```python
from build123d import *

# Parameters (mm, degrees)
SKETCH_2_OUTSIDE_W  = 32.184
SKETCH_2_OUTSIDE_H  = 32.184
CUT_EXTRUDE_1_DEPTH = 59.533728738
CHAMFER_1_SIZE      = 1


with BuildPart() as part:
    # Эскиз1 → Повернуть1 (revolve)
    with BuildSketch(Plane.XY, mode=Mode.PRIVATE) as revolve_1_sk:
        Polygon((-6.58, 0), (-6.58, 8.85), (0, 8.85), (0, 7.448974596), (0.6, 7.288205081), (0.6, 5), (50.6, 5), (50.6, 0), align=None)
    revolve(revolve_1_sk.sketch.rotate(Axis((-1000, 0, 0), (1, 0, 0)), 90), axis=Axis((-1000, 0, 0), (1, 0, 0)))

    # Эскиз2 outside → Вырез-Вытянуть1 (cut, through all)
    with BuildSketch(Plane.ZY.offset(6.58)):
        Rectangle(SKETCH_2_OUTSIDE_W, SKETCH_2_OUTSIDE_H)
        Polygon((0, -8.85), (7.664324823, -4.425), (7.664324823, 4.425), (0, 8.85), (-7.664324823, 4.425), (-7.664324823, -4.425), align=None, mode=Mode.SUBTRACT)
    extrude(amount=-CUT_EXTRUDE_1_DEPTH, mode=Mode.SUBTRACT)

    # Эскиз4 → Вырез-Повернуть1 (revolve, cut)
    with BuildSketch(Plane.XY):
        Polygon((-6.58, 8.075), (-6.297923068, 8.85), (-6.58, 8.85), align=None)
    revolve(axis=Axis((-1000, 0, 0), (1, 0, 0)), mode=Mode.SUBTRACT)

    # Фаска1
    chamfer_1_edges = [part.edges().sort_by_distance(p)[0] for p in [
        (50.6, 0, -5),
    ]]
    chamfer(chamfer_1_edges, length=CHAMFER_1_SIZE)


solid = part.part
```
Geometry: final body of the model. Coordinates: model frame, mm. A direction names the side the tool comes from. Coordinates: 2 decimals unless noted, no trailing zeros. Order: outer loops, then holes, each group sorted by start corner. A loop starts at its lowest first (then second) coordinate and runs counter-clockwise, first axis right, second up. Notation, with made-up numbers: M 36,-39.5 L 83,-39.5 A18 cw 83,-35.5 Z; hole C 44.25,84 d3. An arc over 180 degrees is marked long. Answer in a Markdown table with one row per item. Add a question column.
Q1. Reachability of faces 1 (the flat face through (0.6, 5, -2)), 2 (the conical face through (-6.5, -4.13, 7.2)) from +Z, -Z, +X, -X, +Y, -Y: full face, straight path, thin tool, end or side. Return the list, or none.
Q2. Section query A-A on y = 0. Return the cut outline in (x, z).
Q3. Contact query for flat-ended pins moving along their axis: P1, Ø5, axis at x = 27, z = 6, coming from the +Y side; P2, Ø10, axis at x = 32.5, y = 3.5, coming from the -Z side; P3, Ø10, axis at x = 20.5, y = 4, coming from the +Z side. Output: stop coordinate, or through.
Q4. Section query B-B on x = 8.5. Return the cut outline in (y, z), and give its area (3 significant figures).
Q5. Line query: L1, parallel to Z at x = 13, y = -3; L2, parallel to X at y = -1.25, z = -5.25; L3, parallel to X at y = 5.5, z = -5.5. Output: solid intervals per line, ascending.
Completed:
| question | item | result |
|---|---|---|
| 1 | face 1 | +X |
| 1 | face 2 | +Z, -X, -Y |
| 2 | outline | M -6.58,-7.66 L 0,-7.66 L 0,-7.45 L 0.6,-7.29 L 0.6,-5 L 49.6,-5 L 50.6,-4 L 50.6,4 L 49.6,5 L 0.6,5 L 0.6,7.29 L 0,7.45 L 0,7.66 L -6.58,7.66 Z |
| 3 | P1 | stops at y = 3.57 |
| 3 | P2 | stops at z = -5 |
| 3 | P3 | stops at z = 5 |
| 4 | outline | C 0,0 d10 |
| 4 | area | 78.5 mm2 |
| 5 | L1 | z = -4 to 4 |
| 5 | L2 | x = -6.58 to 0.6 |
| 5 | L3 | x = -6.58 to 0 |
